Source: CAD feature listing. Evaluate the final solid. Frame: model axes, mm. Coordinates: 2 decimals unless noted, no trailing zeros. Order: outer loops, then holes, each group sorted by start corner. A loop starts at its lowest first (then second) coordinate and runs counter-clockwise, first axis right, second up.
Autodesk Inventor part; units mm, degrees
ref_plane "YZ Plane" through (0, 0, 0) normal (1, 0, 0) x (0, 1, 0)
ref_plane "XZ Plane" through (0, 0, 0) normal (0, 1, 0) x (-1, 0, 0)
ref_plane "XY Plane" through (0, 0, 0) normal (0, 0, 1) x (1, 0, 0)
sketch "Sketch1" plane through (0, 0, 0) normal (0, 0, 1) x (1, 0, 0)
  line L0 (38, 290) -> (0, 290)
  line L1 (0, 290) -> (0, 205.5)
  line L2 (0, 205.5) -> (0, 0) construction
  line L3 (0, 0) -> (38, 0) construction
  line L4 (38, 290) -> (38, 205.5)
  line L5 (38, 205.5) -> (0, 205.5)
  line L6 (38, 205.5) -> (38, 0) construction
  dimension "d0" = 580
  dimension "d1" = 38
  dimension "d5" = 411
revolve "Revolution1" add sketch "Sketch1" angle 360 about axis through (0, 0, 0) along (1, 0, 0)
sketch "Sketch2" plane through (0, 0, 0) normal (-1, 0, 0) x (0, 0, 1)
  circle A0 centre (0, 0) radius 205.5
  line L0 (0, 262.5) -> (0, 0) construction
  circle A1 centre (0, 0) radius 290
  circle A2 centre (0, 0) radius 262.5 construction
  line L1 (0, 0) -> (51.2112, 257.4561) construction
  circle A3 centre (51.2112, 257.4561) radius 15
  dimension "d6" = 30
  dimension "d7" = 262.5
  dimension "d8" = 11.25
extrude "Extrusion1" cut sketch "Sketch2" against normal through all contours A3
pattern_circular "Circular Pattern1" count 16 over 360 about axis through (19, 0, 0) along (1, 0, 0) of "Extrusion1"
equation "\"d6\" = dd2"
equation "\"d7\" = 0.5 * k"
equation "\"d0\" = D"
equation "\"d1\" = b"
equation "\"d5\" = dd5"
equation "\"b\" = 38"
equation "\"D\" = 580"
equation "\"k\" = 525"
equation "\"dd2\" = 30"
equation "\"dd5\" = 411"
equation "\"Size_Designation\" = 1.2345"
properties part number "DIN EN 1092-1 Plate Flange for Welding Type 01 - PN 16 400 x 406.4(1)" material "Steel"
Q1. Pin query (flat end, axial travel): P1, Ø5, axis at x = 26, y = 223.5, coming from the +Z side; P2, Ø10, axis at x = 16.5, z = 168.5, coming from the +Y side; P3, Ø18, axis at y = 218.26, z = -145.84, coming from the +X side; P4, Ø5, axis at x = 21, z = 22, coming from the -Y side. Return the tip coordinate at first contact, or that it passes through.
Solutions:
P1: stops at z = 187.77
P2: stops at y = 239.52
P3: passes through
P4: stops at y = -289.34
Q2. Material intervals for line 1 along Z through (x, y) = (21, 132); line 2 along Z through (x, y) = (15, 0); line 3 along Y through (x, z) = (34.5, -4), sorted ascending.
Solutions:
line 1: z = -258.22 to -224.05, -212.47 to -157.5, 157.5 to 212.47, 224.05 to 258.22
line 2: z = -290 to -205.5, 205.5 to 290
line 3: y = -289.97 to -205.46, 205.46 to 289.97
Q3. Pull-direction query (Y, two-part tool) for faces 1 (the flat face through (38, 85, -192)), 2 (the cylindrical face through (18.734, 48.601, 272.227)), 3 (the cylindrical face through (18.734, 276.608, -87.108)); classes: pulls with the +Y half, pulls with the -Y half, needs draft (parallel to the pull), parting line crosses it, or undercut.
Solutions:
face 1: needs draft
face 2: undercut
face 3: parting line crosses it
Q4. Section query A-A on y = 0. Output: boundary loops of the cut face in (x, z), plus the area to 3 significant figures.
Solutions:
outline: (0, -290) - (38, -290) - (38, -205.5) - (0, -205.5) - close; (0, 205.5) - (38, 205.5) - (38, 290) - (0, 290) - close
area: 6,420 mm2
